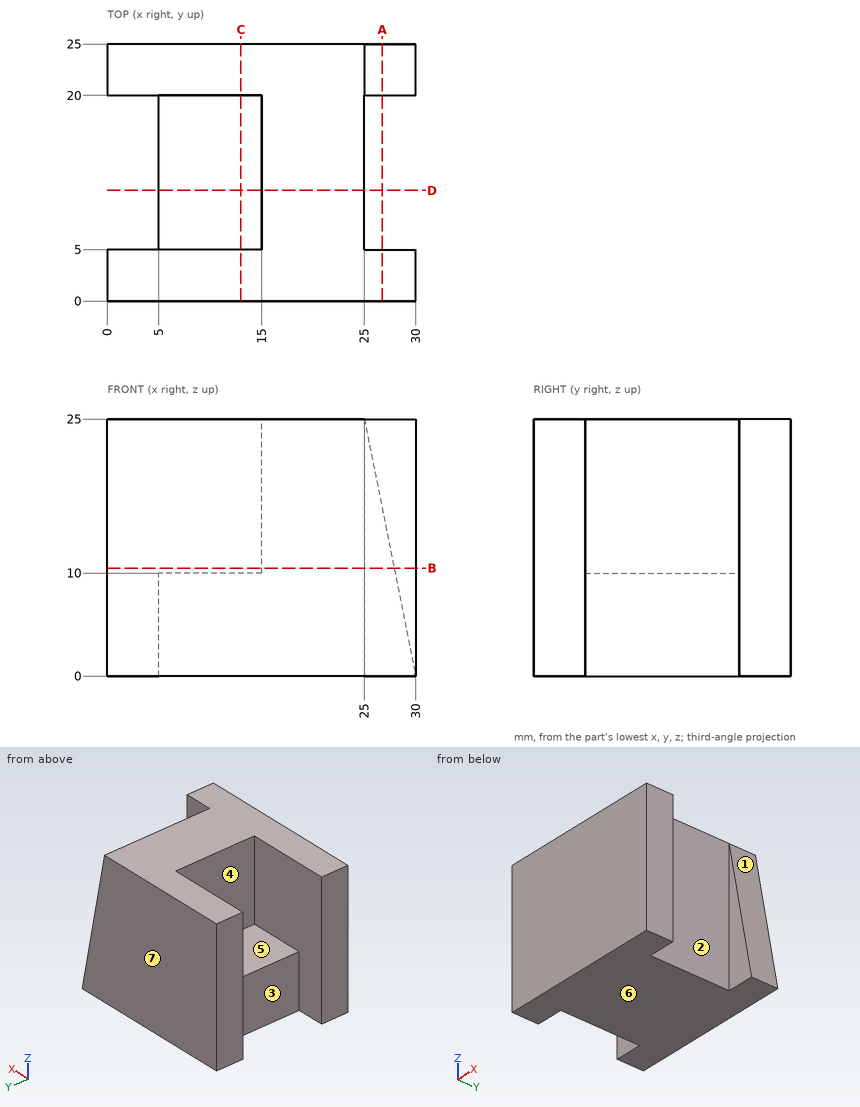
Input: dimensioned drawing with shaded views. Units: mm. Origin: part minimum x, y, z. A direction names the side the tool comes from. Coordinates: 2 decimals unless noted, no trailing zeros. Order: outer loops, then holes, each group sorted by start corner. A loop starts at its lowest first (then second) coordinate and runs counter-clockwise, first axis right, second up.
(1) Section query C-C (x = 13). Return the cut outline in (y, z).
(2) Section query B-B (z = 10.5). Return the cut outline in (x, y).
(3) First-contact query: pin 1 (7.5 mm diameter, centred on y = 12.5, z = 19, fed in from -X); pin 2 (1 mm diameter, centred on y = 15, z = 19.5, fed in from +X); pin 3 (5 mm diameter, centred on y = 10.5, z = 5.5, fed in from -X). Flat tips, straight axial feed; report the tip coordinate or a pass-through.
(4) Access query for the marked faces 1, 2, 3 and 4. Directions: +Z, -Z, +X, -X, +Y, -Y. A direction counts if a zero-diameter tool reaches every point of the face in a straight line with its end or side. Return the directions, or none.
(5) Section query D-D (y = 10.75). Return the cut outline in (x, z).
(6) Draft query along Y for the marked faces 5, 6 and 7. Return one class per face: pulls with the +Y half, pulls with the -Y half, needs draft (parallel to the pull), parting line crosses it, or undercut.
(7) Material intervals for probe 1 along Y at (x, z) = (1.75, 23.5); probe 2 along X at (y, z) = (12, 13.5); probe 3 along X at (y, z) = (12, 2.5), sorted ascending.
(8) Section query A-A (x = 26.75). Return the cut outline in (y, z), plus the area to 3 significant figures.
Solution:
1. outline: (0, 0) - (25, 0) - (25, 25) - (20, 25) - (20, 10) - (5, 10) - (5, 25) - (0, 25) - close
2. outline: (0, 0) - (30, 0) - (30, 5) - (25, 5) - (25, 20) - (27.9, 20) - (27.9, 25) - (0, 25) - (0, 20) - (15, 20) - (15, 5) - (0, 5) - close
3. pin 1: stops at x = 15
3. pin 2: stops at x = 25
3. pin 3: stops at x = 5
4. face 1: +Z, +X, +Y
4. face 2: +Z, -Z, +X
4. face 3: +Z, -Z, -X
4. face 4: +Z, -X
5. outline: (5, 0) - (25, 0) - (25, 25) - (15, 25) - (15, 10) - (5, 10) - close
6. face 5: undercut
6. face 6: needs draft
6. face 7: pulls with the +Y half
7. probe 1: y = 0 to 5, 20 to 25
7. probe 2: x = 15 to 25
7. probe 3: x = 5 to 25
8. outline: (0, 0) - (5, 0) - (5, 25) - (0, 25) - close; (20, 0) - (25, 0) - (25, 16.25) - (20, 16.25) - close
8. area: 206 mm2
